The figure shows three views and two pictorial views of one solid part (mm, origin at its lowest corner). Answer the questions. Round coordinates to 2 decimals unless told otherwise and drop trailing zeros. Write each loop counter-clockwise with the first axis right and the second up, starting at its lowest first coordinate (ties: lowest second). Pieces come first, ordered by that corner, then holes. Notation, with made-up numbers: M 3.5,80 L 31.5,80 A14 cw 31.5,103 Z; hole C 33.5,30 d2. An arc over 180 degrees is marked long. One line per item, written item: value. Start each with the question number.
Q1. Find section D-D (z = 33). Write down the section's boundary in (x, y).
Q2. Given pin 1 Ø5 at (x, y) = (54.5, 44) entering from -Z; pin 2 Ø10 at (x, z) = (22, 39.5) entering from +Y; pin 3 Ø4 at (y, z) = (74, 71.5) entering from +X; pin 4 Ø10 at (x, z) = (38, 14.5) entering from +Y, each flat-ended and moving along its own axis, determine where each tip first touches the part or whether it passes through.
Q3. Find section A-A (x = 70). Write down the section's boundary in (y, z), and give its area (3 significant figures).
Q4. Find section B-B (z = 58.5). Write down the section's boundary in (x, y).
Q5. Consider probe 1 along Y at (x, z) = (70, 44); probe 2 along Y at (x, z) = (83.5, 68); probe 3 along X at (y, z) = (72, 49). Determine where each line is inside the solid, lowest interval first.
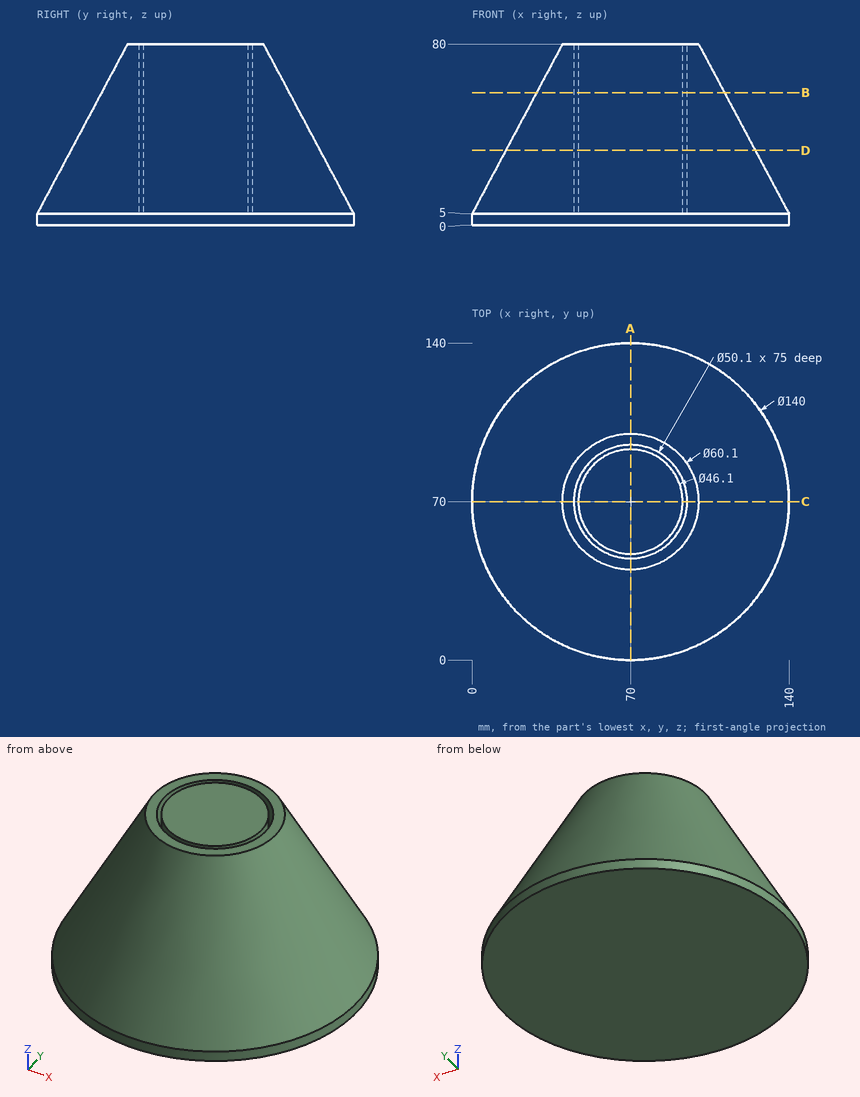
The answers:
1. outline: C 70,70 d110.17; C 70,70 d46.1; hole C 70,70 d50.1
2. pin 1: z = 0
2. pin 2: y = 99.96
2. pin 3: x = 105.44
2. pin 4: y = 130.48
3. outline: M 0,0 L 140,0 L 140,5 L 100.05,80 L 95.05,80 L 95.05,5 L 93.05,5 L 93.05,80 L 46.95,80 L 46.95,5 L 44.95,5 L 44.95,80 L 39.95,80 L 0,5 Z
3. area: 7,900 mm2
4. outline: C 70,70 d83; C 70,70 d46.1; hole C 70,70 d50.1
5. probe 1: 20.77 to 44.95, 46.95 to 93.05, 95.05 to 119.23
5. probe 2: 36.15 to 48.9, 51.32 to 88.68, 91.1 to 103.85
5. probe 3: 23.48 to 45.03, 47.04 to 92.96, 94.97 to 116.52
